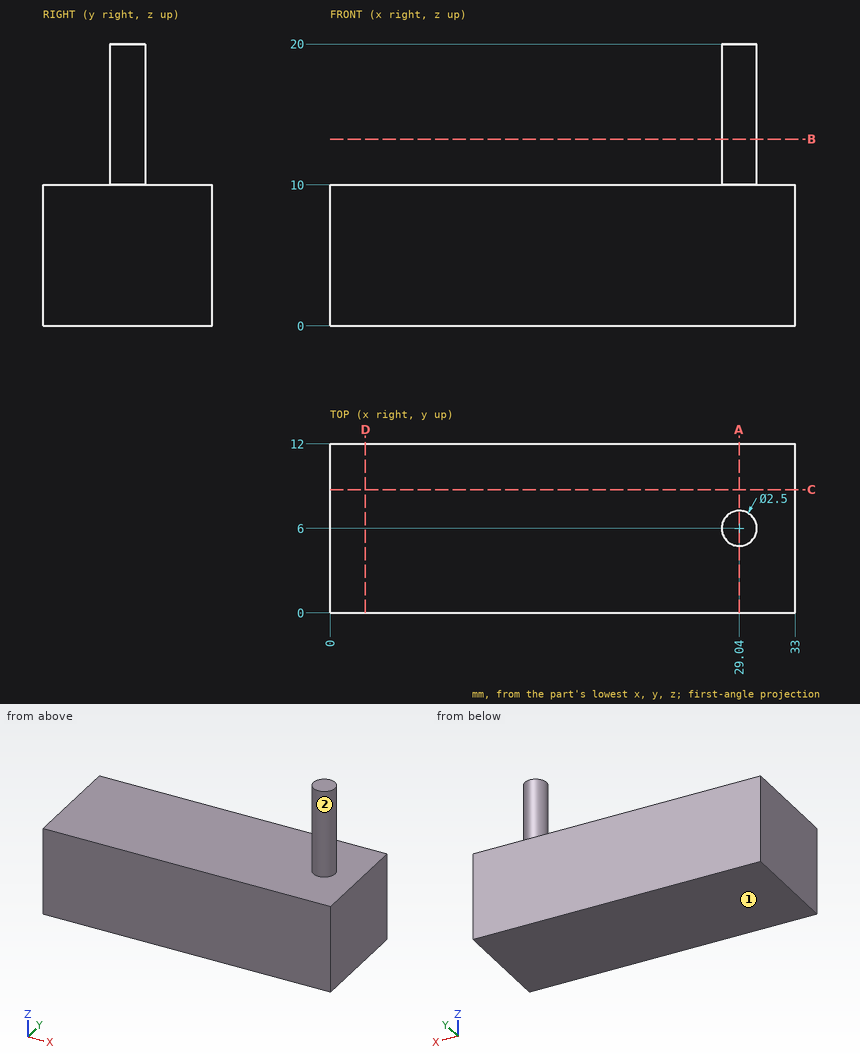
Drawing for the job (mm, zero at the part's lowest x, y, z). A direction names the side the tool comes from. Coordinates: 2 decimals unless noted, no trailing zeros. Order: outer loops, then holes, each group sorted by start corner. A loop starts at its lowest first (then second) coordinate and runs counter-clockwise, first axis right, second up.
Item 1: 3-axis set-ups, long thin cutter, end or side, ignore diameter. For the marked faces 1 and 2: which of +Z, -Z, +X, -X, +Y, -Y reach the whole face in a straight line?
Check sheet entries:
face 1: -Z, +X, -X, +Y, -Y
face 2: +Z
Item 2: Pin check, flat tip, straight feed: pin 1 Ø6 at (x, z) = (14.5, 14.5) entering from -Y. Stop position of the tip, or through.
Check sheet entries:
pin 1: passes through
Item 3: Band-saw the part on B-B on z = 13.25. List the corners of the cut face in (x, y).
Check sheet entries:
outline: circle Ø2.5 at (29.04, 6)
Item 4: Band-saw the part on A-A on x = 29.04. List the corners of the cut face in (y, z).
Check sheet entries:
outline: (0, 0) - (12, 0) - (12, 10) - (7.25, 10) - (7.25, 20) - (4.75, 20) - (4.75, 10) - (0, 10) - close
Item 5: Band-saw the part on C-C on y = 8.75. List the corners of the cut face in (x, z).
Check sheet entries:
outline: (0, 0) - (33, 0) - (33, 10) - (0, 10) - close
Item 6: Drill centre lines: L1, parallel to Z at x = 17.5, y = 10; L2, parallel to X at y = 5.5, z = 10.75. Where is each one in solid material? Low to high.
Check sheet entries:
L1: z = 0 to 10
L2: x = 27.89 to 30.19
Item 7: Band-saw the part on D-D on x = 2.5. List the corners of the cut face in (y, z), plus the area to 3 significant figures.
Check sheet entries:
outline: (0, 0) - (12, 0) - (12, 10) - (0, 10) - close
area: 120 mm2
